Could you check a few things on this model? Use its own coordinates, in mm. A direction names the side the tool comes from. Give positions to 0.01 mm unless a question says otherwise; leave off trailing zeros. Loops run counter-clockwise (first coordinate to the right, second up) from the corner with the lowest first, then second, coordinate; pieces in that order, holes last. Notation, with made-up numbers: (58.25, 54) -> (98.25, 54) arc R7 ccw to (98.25, 61) -> close; hole circle Ø7 at (-39, 77.25). An arc over 180 degrees is marked (long way). Put each result on its own line as item: value.
```python
from build123d import *

# Parameters (mm, degrees)
SKETCH_1_R               = 10
SKETCH_1_R_2             = 3
SKETCH_1_R_3             = 1.5
EXTRUDE_1_DEPTH          = 3
SKETCH_2_R               = 4
EXTRUDE_2_DEPTH          = 16
SKETCH_6_R               = 6
EXTRUDE_3_DEPTH          = 12
CUT_EXTRUDE_1_DEPTH      = 32.368774283
CUT_EXTRUDE_1_DEPTH_BACK = 32.368774283
SKETCH_5_R               = 1.5
CUT_EXTRUDE_3_DEPTH      = 32.368774372
CUT_EXTRUDE_3_DEPTH_BACK = 32.368774372
SKETCH_7_R               = 1.5


with BuildPart() as part:
    # Sketch 1 → Extrude 1 (new body)
    with BuildSketch(Plane(origin=(0, 0, 0), x_dir=(1, 0, 0), z_dir=(0, 1, 0))):
        with Locations(Location((0, 0, 0), (0, 0, 270))):
            Circle(SKETCH_1_R)
        with Locations(Location((0, 0, 0), (0, 0, 270))):
            Circle(SKETCH_1_R_2, mode=Mode.SUBTRACT)
        with Locations(Location((0, 7, 0), (0, 0, 270))):
            Circle(SKETCH_1_R_3, mode=Mode.SUBTRACT)
        with Locations(Location((7, 0, 0), (0, 0, 270))):
            Circle(SKETCH_1_R_3, mode=Mode.SUBTRACT)
        with Locations(Location((0, -7, 0), (0, 0, 270))):
            Circle(SKETCH_1_R_3, mode=Mode.SUBTRACT)
        with Locations(Location((-7, 0, 0), (0, 0, 270))):
            Circle(SKETCH_1_R_3, mode=Mode.SUBTRACT)
    extrude(amount=EXTRUDE_1_DEPTH)

    # Sketch 2 → Extrude 2 (add)
    with BuildSketch(Plane(origin=(0, 0, 0), x_dir=(1, 0, 0), z_dir=(0, 1, 0))):
        with Locations(Location((0, 0, 0), (0, 0, 270))):
            Circle(SKETCH_2_R)
    extrude(amount=EXTRUDE_2_DEPTH)

    # Sketch 6 → Extrude 3 (add)
    with BuildSketch(Plane(origin=(0, 16, 0), x_dir=(1, 0, 0), z_dir=(0, 1, 0))):
        with Locations(Location((0, 0, 0), (0, 0, 270))):
            Circle(SKETCH_6_R)
    extrude(amount=EXTRUDE_3_DEPTH)

    # Sketch 5 → Cut-Extrude 1 (cut, two sides: drawn at the far end of the back side and taken through both)
    with BuildSketch(Plane(origin=(0, 0, 0), x_dir=(0, 1, 0), z_dir=(0.7071067811865438, 0, -0.7071067811865512)).offset(-CUT_EXTRUDE_1_DEPTH_BACK)):
        with Locations(Location((20, 0, 0), (0, 0, 270))):
            Circle(SKETCH_5_R)
    extrude(amount=CUT_EXTRUDE_1_DEPTH + CUT_EXTRUDE_1_DEPTH_BACK, mode=Mode.SUBTRACT)

    # Sketch 7 → Cut-Extrude 3 (cut, two sides: drawn at the far end of the back side and taken through both)
    with BuildSketch(Plane(origin=(0, 0, 0), x_dir=(0, 1, 0), z_dir=(-0.7071067811865537, 0, -0.7071067811865414)).offset(-CUT_EXTRUDE_3_DEPTH_BACK)):
        with Locations(Location((24, 0, 0), (0, 0, 270))):
            Circle(SKETCH_7_R)
    extrude(amount=CUT_EXTRUDE_3_DEPTH + CUT_EXTRUDE_3_DEPTH_BACK, mode=Mode.SUBTRACT)


solid = part.part
```
1. For faces 4 (the face through (0.1, 3, 4.3)), 5 (the face through (-5.323, 21.916, 2.769)), 6 (the face through (5.536, 1.479, -0.325)), 7 (the face through (0, 28, 0)), 8 (the face through (-9.76, 1.48, -2.17)), which set-ups out of +Z, -Z, +X, -X, +Y, -Y let a thin tool reach every point of the face, with its end or its side?
Recorded:
face 4: none
face 5: +Y
face 6: -Y
face 7: +Z, -Z, +X, -X, +Y
face 8: +Y, -Y
2. If we section it at A-A (x = -7.5): List the corners of the cut face in (y, z) for me, then the cut area to 3 significant figures.
Recorded:
outline: (0, -6.61) -> (3, -6.61) -> (3, -1.41) -> (0, -1.41) -> close; (0, 1.41) -> (3, 1.41) -> (3, 6.61) -> (0, 6.61) -> close
area: 31.2 mm^2
3. I'm going to push flat-ended pins straight in: pin 1 (4 mm diameter, centred on x = -2.5, y = 10.5, fed in from -Z); pin 2 (2.5 mm diameter, centred on x = -7, z = 0, fed in from -Y); pin 3 (2 mm diameter, centred on x = 4, y = 16.5, fed in from +Z); pin 4 (9.5 mm diameter, centred on x = 0.5, z = -0.5, fed in from -Y). Where does each tip first touch, or does it pass through?
Recorded:
pin 1: stops at z = -3.97
pin 2: stops at y = 16
pin 3: stops at z = 5.2
pin 4: stops at y = 0
4. I need wall thicknesses on line 1 (X direction, y = 1.55, z = 0); line 2 (Y direction, x = -4.25, z = -7.25); line 3 (X direction, y = 2.05, z = 7). Which ranges of each line are inside material? Lowest first, please.
Recorded:
line 1: x = -10 to -8.5, -5.5 to 5.5, 8.5 to 10
line 2: y = 0 to 3
line 3: x = -7.14 to -1.5, 1.5 to 7.14
5. If we section it at B-B (z = -7): List the corners of the cut face in (x, y) for me, then the cut area to 3 significant figures.
Recorded:
outline: (-7.14, 0) -> (-1.5, 0) -> (-1.5, 3) -> (-7.14, 3) -> close; (1.5, 0) -> (7.14, 0) -> (7.14, 3) -> (1.5, 3) -> close
area: 33.8 mm^2
6. If we section it at C-C (y = 14.75): List the corners of the cut face in (x, z) for me, then the cut area to 3 significant figures.
Recorded:
outline: circle Ø8 at (0, 0)
area: 50.3 mm^2
7. Thinking about a two-plate mould opening in Y: for faces 1 (the face through (-3.92, 16, -1.42)), 2 (the face through (0.07, 1.48, -8.5)), 3 (the face through (0, 0, 0)), which applies, pulls with the +Y half, pulls with the -Y half, needs draft (parallel to the pull), parting line crosses it, or undercut?
Recorded:
face 1: undercut
face 2: needs draft
face 3: pulls with the -Y half
8. If we section it at D-D (z = 0): Count the separate pieces of the cut face and the enclosed holes in it, then the cut area to 3 significant figures.
Recorded:
separate pieces: 3
enclosed holes: 2
area: 270 mm^2
